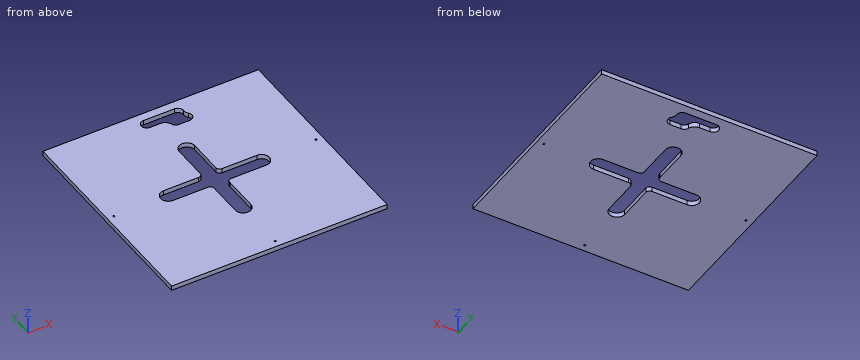
from build123d import *

# Parameters (mm, degrees)
CROQUIS1_W                   = 277
CROQUIS1_H                   = 275
BRIDA_BASE1_DEPTH            = 6
CORTAR_EXTRUIR4_DEPTH        = 10
REDONDEO2_R                  = 10
TALADRO_DE_MARGEN_PARA_M21_D = 2.4
CORTAR_EXTRUIR5_DEPTH        = 196.254961669
MATRIZC1_COUNT               = 4
REDONDEO3_R                  = 5


# Sheet-metal steps are written as plain solids
with BuildPart() as part:
    # Croquis1 → Brida base1 (new body)
    with BuildSketch(Plane.XY):
        Rectangle(CROQUIS1_W, CROQUIS1_H)
    extrude(amount=-BRIDA_BASE1_DEPTH)

    # Croquis6 → Cortar-Extruir4 (cut)
    with BuildSketch(Plane(origin=(0, 0, -6), x_dir=(-1, 0, 0), z_dir=(0, 0, -1))):
        with BuildLine():
            Line((-9.101020514, 112.5), (16, 112.5))
            ThreePointArc((16, 112.5), (23, 119.5), (16, 126.5))
            Line((16, 126.5), (-24, 126.5))
            ThreePointArc((-24, 126.5), (-30.494583009, 122.111587935), (-28.846049894, 114.448683298))
            ThreePointArc((-28.846049894, 114.448683298), (-28.423802379, 114.487159047), (-28, 114.5))
            Line((-28, 114.5), (-14, 114.5))
            ThreePointArc((-14, 114.5), (-11.354248689, 113.980740698), (-9.101020514, 112.5))
        make_face()
        with BuildLine():
            ThreePointArc((-14, 100.5), (-7.519259302, 104.854248689), (-9.101020514, 112.5))
            Line((-9.101020514, 112.5), (-24, 112.5))
            ThreePointArc((-24, 112.5), (-26.611587935, 113.005416991), (-28.846049894, 114.448683298))
            ThreePointArc((-28.846049894, 114.448683298), (-34.987159047, 107.076197621), (-28, 100.5))
            Line((-28, 100.5), (-14, 100.5))
        make_face()
        with BuildLine():
            Line((-24, 112.5), (-9.101020514, 112.5))
            ThreePointArc((-9.101020514, 112.5), (-11.354248689, 113.980740698), (-14, 114.5))
            Line((-14, 114.5), (-28, 114.5))
            ThreePointArc((-28, 114.5), (-28.423802379, 114.487159047), (-28.846049894, 114.448683298))
            ThreePointArc((-28.846049894, 114.448683298), (-26.611587935, 113.005416991), (-24, 112.5))
        make_face()
    extrude(amount=-CORTAR_EXTRUIR4_DEPTH, mode=Mode.SUBTRACT)

    # Redondeo2
    redondeo2_edges = [part.edges().sort_by_distance(p)[0] for p in [
        (28.846049894, 114.448683298, -3),
        (9.101020514, 112.5, -3),
    ]]
    fillet(redondeo2_edges, radius=REDONDEO2_R)

    # Taladro de margen para M21 (through all)
    with Locations(Plane(origin=(0, 0, -6), x_dir=(-1, 0, 0), z_dir=(0, 0, -1))):
        with Locations((-130, 0), (130, 0), (0, -129)):
            Hole(TALADRO_DE_MARGEN_PARA_M21_D / 2)

    # Croquis16 → Cortar-Extruir5 (cut, through all)
    with BuildSketch(Plane(origin=(0, 0, -6), x_dir=(-1, 0, 0), z_dir=(0, 0, -1))):
        with BuildLine():
            Line((10, 60), (10, -60))
            ThreePointArc((10, -60), (0, -70), (-10, -60))
            Line((-10, -60), (-10, 60))
            ThreePointArc((-10, 60), (0, 70), (10, 60))
        make_face()
    cortar_extruir5 = extrude(amount=-CORTAR_EXTRUIR5_DEPTH, mode=Mode.SUBTRACT)

    # MatrizC1: Cortar-Extruir5 ×4 about axis
    matrizc1_axis = Axis((0, 0, 0), (0, 0, 1))
    for i in range(1, MATRIZC1_COUNT):
        add(cortar_extruir5.rotate(matrizc1_axis, i * 360 / MATRIZC1_COUNT), mode=Mode.SUBTRACT)

    # Redondeo3
    redondeo3_edges = [part.edges().sort_by_distance(p)[0] for p in [
        (10, 10, -3),
        (10, -10, -3),
        (-10, 10, -3),
        (-10, -10, -3),
    ]]
    fillet(redondeo3_edges, radius=REDONDEO3_R)


solid = part.part
The model under review builds one solid part; all positions refer to its coordinate system, in mm. Give positions to 0.01 mm unless a question says otherwise; leave off trailing zeros. Write each loop counter-clockwise with the first axis right and the second up, starting at its lowest first coordinate (ties: lowest second). Pieces come first, ordered by that corner, then holes.
1. Add section B-B, the plane z = -2.5. Count the separate pieces of the cut face and the enclosed holes in it, plus the area to 3 significant figures.
2. Add section A-A, the plane y = 38. Write out the cut boundary in (x, z).
3. Wall thickness on L1, parallel to X at y = 53, z = -0.5; L2, parallel to Y at x = -42, z = -0.25; L3, parallel to Y at x = 33, z = -2.25: over which ranges is each line inside the solid? List them lowest first.
Worked answers:
1. separate pieces: 1
1. enclosed holes: 5
1. area: 70,100 mm2
2. outline: (-138.5, -6) - (-10, -6) - (-10, 0) - (-138.5, 0) - close; (10, -6) - (138.5, -6) - (138.5, 0) - (10, 0) - close
3. L1: x = -138.5 to -10, 10 to 138.5
3. L2: y = -137.5 to -10, 10 to 137.5
3. L3: y = -137.5 to -10, 10 to 102.6, 112.45 to 137.5
